from build123d import *

# Parameters (mm, degrees)
DODANIE_WYCI_GNI_CIE1_DEPTH = 5
SZKIC3_R                    = 3
WYTNIJ_WYCI_GNI_CIE1_DEPTH  = 5


with BuildPart() as part:
    # Szkic1 → Dodanie-wyciągnięcie1 (new body)
    with BuildSketch(Plane.XY):
        with BuildLine():
            Line((-100, 0), (0, 0))
            Line((0, 0), (0, 170))
            Line((0, 170), (-102.948040342, 170))
            ThreePointArc((-102.948040342, 170), (-115.328169963, 165.707717548), (-122.394398271, 154.673239056))
            ThreePointArc((-122.394398271, 154.673239056), (-126.526512484, 134.017204351), (-129.061437885, 113.105))
            ThreePointArc((-129.061437885, 113.105), (-128.631920304, 63.328972076), (-119.214524038, 14.4500391))
            ThreePointArc((-119.214524038, 14.4500391), (-112.020831544, 4.015644868), (-100, 0))
        make_face()
        with BuildLine():
            ThreePointArc((-103.503346853, 80.578026571), (-100.574414665, 87.649094383), (-93.503346853, 90.578026571))
            Line((-93.503346853, 90.578026571), (-79.671539283, 90.578026571))
            ThreePointArc((-79.671539283, 90.578026571), (-72.600471471, 87.649094383), (-69.671539283, 80.578026571))
            Line((-69.671539283, 80.578026571), (-69.671539283, 32.262674049))
            ThreePointArc((-69.671539283, 32.262674049), (-86.587443068, 15.346770264), (-103.503346853, 32.262674049))
            Line((-103.503346853, 32.262674049), (-103.503346853, 80.578026571))
        make_face(mode=Mode.SUBTRACT)
        with BuildLine():
            Line((-103.503346853, 120.578026571), (-103.557564737, 139.250268571))
            ThreePointArc((-103.557564737, 139.250268571), (-100.443696898, 145.391700798), (-93.636751398, 146.430380577))
            Line((-93.636751398, 146.430380577), (-74.144065049, 139.891934241))
            ThreePointArc((-74.144065049, 139.891934241), (-70.835961623, 137.44494736), (-69.590709059, 133.523131566))
            Line((-69.590709059, 133.523131566), (-69.657118792, 110.563564309))
            ThreePointArc((-69.657118792, 110.563564309), (-71.126680855, 107.037383175), (-74.657097877, 105.578026571))
            Line((-74.657097877, 105.578026571), (-88.503346853, 105.578026571))
            ThreePointArc((-88.503346853, 105.578026571), (-99.109948571, 109.971424853), (-103.503346853, 120.578026571))
        make_face(mode=Mode.SUBTRACT)
    dodanie_wyci_gni_cie1 = extrude(amount=DODANIE_WYCI_GNI_CIE1_DEPTH)

    # Lustro1: Dodanie-wyciągnięcie1 across plane
    add(dodanie_wyci_gni_cie1.mirror(Plane(origin=(0, 0, 5), x_dir=(0, 0, 1), z_dir=(-1, 0, 0))))

    # Szkic3 → Wytnij-wyciągnięcie1 (cut)
    with BuildSketch(Plane.XY.offset(5)):
        with Locations((0, 73.388617168)):
            Circle(SZKIC3_R)
        with Locations((-21.955, 111.415792648)):
            Circle(SZKIC3_R)
        with Locations((21.955, 111.415792648)):
            Circle(SZKIC3_R)
    extrude(amount=-WYTNIJ_WYCI_GNI_CIE1_DEPTH, mode=Mode.SUBTRACT)


solid = part.part
Read the model definition and answer for the solid it produces. Units are mm, in the model's axes. A direction names the side the tool comes from. Coordinates: 2 decimals unless noted, no trailing zeros. Write each loop counter-clockwise with the first axis right and the second up, starting at its lowest first coordinate (ties: lowest second). Pieces come first, ordered by that corner, then holes. Notation, with made-up numbers: (-34.75, 37.25) - (0.25, 37.25) arc R30 cw to (0.25, 67.25) - close; hole circle Ø1 at (11.5, 73.25). An arc over 180 degrees is marked (long way). One line per question, with ' | ' between items.
Q1. Determine the mould class of faces 1 (the cylindrical face through (-86.22, 15.35, 2.46)), 2 (the flat face through (1, 0, 2)), 3 (the cylindrical face through (-100.65, 87.57, 2.46)), 4 (the flat face through (2, 86, 0)) for opening direction Y: +Y half, -Y half, draft (parallel to the pull), parting line (faces both ways), or undercut.
Result set:
face 1: undercut | face 2: -Y half | face 3: undercut | face 4: draft
Q2. Consider L1, parallel to X at y = 68, z = 2.6; L2, parallel to X at y = 48.5, z = 1.25; L3, parallel to Y at x = 83.5, z = 3.85. Determine where each line is inside the solid, lowest interval first. Write a range as [from, to].
Result set:
L1: [-129.06, -103.5], [-69.67, 69.67], [103.5, 129.06] | L2: [-126.74, -103.5], [-69.67, 69.67], [103.5, 126.74] | L3: [0, 15.63], [90.58, 105.58], [143.03, 170]
Q3. For faces 5 (the cylindrical face through (-70.87, 137.49, 2.46)), 6 (the cylindrical face through (-112, 4, 2)), determine the directions among +Z, -Z, +X, -X, +Y, -Y from which every point of the face is accessible in a straight line to the end or side of a thin tool.
Result set:
face 5: +Z, -Z | face 6: +Z, -Z, -X, -Y
Q4. Find section B-B, the plane y = 18.5. Write down the section's boundary in (x, z).
Result set:
outline: (-120.35, 0) - (-96.42, 0) - (-96.42, 5) - (-120.35, 5) - close; (-76.75, 0) - (76.75, 0) - (76.75, 5) - (-76.75, 5) - close; (96.42, 0) - (120.35, 0) - (120.35, 5) - (96.42, 5) - close
Q5. Each of these flat-tipped pins is pushed along its axis until it touches: P1, Ø3, axis at y = 142.5, z = 3.5, coming from the +X side; P2, Ø2.5, axis at y = 53, z = 2, coming from the +X side. Where does it stop, or does it pass through?
Result set:
P1: x = 125.31 | P2: x = 127.57
Q6. Find section C-C, the plane z = 1.4. State how many separate pieces and enclosed holes the cut face has, plus the area to 3 significant figures.
Result set:
separate pieces: 1 | enclosed holes: 7 | area: 35,200 mm^2
Q7. Find section A-A, the plane x = 0. Write down the section's boundary in (y, z), plus the area to 3 significant figures.
Result set:
outline: (0, 0) - (70.39, 0) - (70.39, 5) - (0, 5) - close; (76.39, 0) - (170, 0) - (170, 5) - (76.39, 5) - close | area: 820 mm^2
